Here's how the part is built. I have some questions about the finished solid (model axes, mm). Coordinates: 2 decimals unless noted, no trailing zeros. Order: outer loops, then holes, each group sorted by start corner. A loop starts at its lowest first (then second) coordinate and runs counter-clockwise, first axis right, second up. Notation, with made-up numbers: (-16, -6.75) - (28, -6.75) arc R22 cw to (28, 29.25) - close; hole circle Ø10 at (51.5, -16.75). An arc over 180 degrees is marked (long way). Answer as CSV lines item,"result". Start each with the question number.
Item 1: Imagine slicing it at C-C on z = 2.5. List the corners of the cut face in (x, y) for me.
Item 2: Imagine slicing it at B-B on x = -2.25. List the corners of the cut face in (y, z) for me, and give its area (3 significant figures).
Item 3: Imagine slicing it at A-A on y = -23. List the corners of the cut face in (x, z) for me, and give its area (3 significant figures).
Item 4: I need wall thicknesses on line 1 (X direction, y = -44, z = 0.25); line 2 (X direction, y = -27, z = 3); line 3 (Z direction, x = 3, y = -51.5). Which ranges of each line are inside material? Lowest first, please.
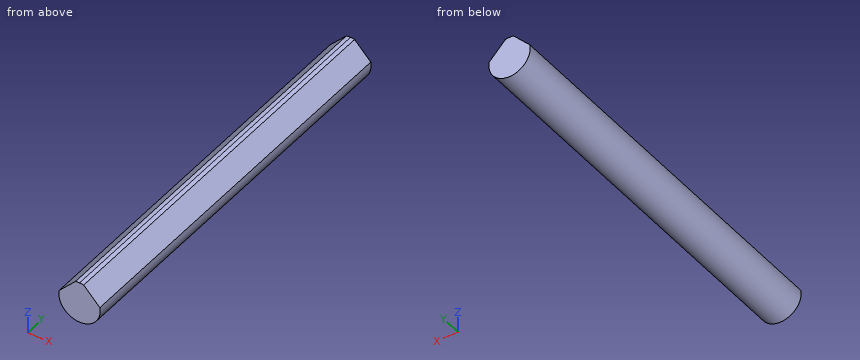
from build123d import *

# Parameters (mm, degrees)
F1_DEPTH = 76.2


with BuildPart() as f1:
    # F0 (on Front) → F1 (new body)
    with BuildSketch(Plane.XZ):
        with BuildLine():
            Line((3.910824, 0.711952), (0.79495, 3.894801))
            ThreePointArc((0.79495, 3.894801), (0.399498, 3.954974), (0, 3.9751))
            ThreePointArc((0, 3.9751), (-0.399498, 3.954974), (-0.79495, 3.894801))
            Line((-0.79495, 3.894801), (-3.910824, 0.711952))
            ThreePointArc((-3.910824, 0.711952), (0, -3.9751), (3.910824, 0.711952))
        make_face()
    extrude(amount=F1_DEPTH)


solid = f1.part
Responses:
1,outline,"(-2.16, -76.2) - (2.16, -76.2) - (2.16, 0) - (-2.16, 0) - close"
2,outline,"(-76.2, -3.28) - (0, -3.28) - (0, 2.41) - (-76.2, 2.41) - close"
2,area,"433 mm^2"
3,outline,"(-3.91, 0.71) arc R3.98 ccw (long way) to (3.91, 0.71) - (0.79, 3.89) arc R3.98 ccw to (0, 3.98) arc R3.98 ccw to (-0.79, 3.89) - close"
3,area,"45.5 mm^2"
4,line 1,"x = -3.97 to 3.97"
4,line 2,"x = -1.67 to 1.67"
4,line 3,"z = -2.61 to 1.64"
